Input: part model. Units: mm. Frame: model coordinates. Face numbers are marked on the shaded views. A direction names the side the tool comes from. Coordinates: 2 decimals unless noted, no trailing zeros. Write each loop counter-clockwise with the first axis right and the second up, starting at its lowest first coordinate (ties: lowest second). Pieces come first, ordered by that corner, then holes. Notation, with made-up numbers: (71.25, 66.25) -> (107.25, 66.25) arc R9 ccw to (107.25, 81.25) -> close; hole circle Ø8 at (-33.75, -35.5). An arc over 180 degrees is marked (long way). Use one line per item in the form item = value. Start each with the question number.
(1) Cut plane C-C on x = 78. Return the cut outline in (y, z), plus the area to 3 significant figures.
(2) Pull-direction query (Y, two-part tool) for the marked faces 6, 7 and 8; classes: released by +Y, released by -Y, zero draft, split by the parting line, or undercut.
(3) Set-up query: the marked faces 1, 2, 3, 4 and 5. Return all of +Z, -Z, +X, -X, +Y, -Y with unobstructed straight access to the full face (end or side cutting, diameter ignored); none if empty.
(4) Cut plane B-B on y = 0. Return the cut outline in (x, z), plus the area to 3 significant figures.
(5) Ray query, line 1 along X through (y, z) = (-13.5, 16); line 2 along X through (y, z) = (11, 10.5); line 3 along Y through (x, z) = (27, -6.5). Return the intervals inside material, ascending.
(6) First-contact query: pin 1 (6 mm diameter, centred on x = 101, y = -14.5, fed in from -Z); pin 2 (10 mm diameter, centred on x = 47.5, y = 1, fed in from +Z); pin 3 (1.5 mm diameter, centred on x = 8, z = 0.5, fed in from -Y); pin 4 (19.5 mm diameter, centred on x = 62.5, z = -3, fed in from +Y). Flat tips, straight axial feed; report the tip coordinate or a pass-through.
(7) Cut plane D-D on y = -7. Return the cut outline in (x, z), plus the area to 3 significant figures.
(8) Cut plane A-A on z = -1.5. Return the cut outline in (x, y), plus the area to 3 significant figures.
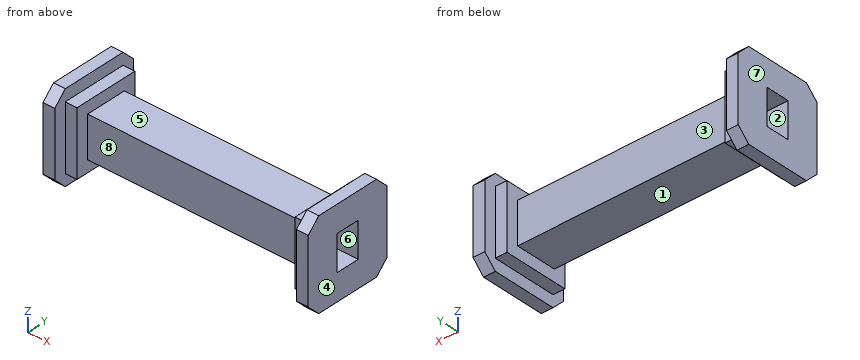
```python
from build123d import *

# Parameters (mm, degrees)
SKETCH1_W           = 38.1
SKETCH1_H           = 38.1
BOSS_EXTRUDE1_DEPTH = 114.3
CUT_EXTRUDE1_START  = -5.08
SKETCH3_W           = 38.1
SKETCH3_H           = 38.1
SKETCH3_W_2         = 27.94
SKETCH3_H_2         = 27.94
CUT_EXTRUDE1_DEPTH  = 104.14
CUT_EXTRUDE2_START  = -93.98
SKETCH4_W           = 38.1
SKETCH4_H           = 38.1
SKETCH4_W_2         = 17.78
SKETCH4_H_2         = 17.78
CUT_EXTRUDE2_DEPTH  = 93.98
SKETCH5_W           = 15.24
SKETCH5_H           = 10.16
CUT_EXTRUDE3_DEPTH  = 118.432086757
CHAMFER1_SIZE       = 5.08


with BuildPart() as part:
    # Sketch1 → Boss-Extrude1 (new body)
    with BuildSketch(Plane(origin=(0, 0, 0), x_dir=(0, 0, -1), z_dir=(1, 0, 0))):
        Rectangle(SKETCH1_W, SKETCH1_H)
    extrude(amount=BOSS_EXTRUDE1_DEPTH)

    # Sketch3 → Cut-Extrude1 (cut)
    with BuildSketch(Plane.ZY.offset(CUT_EXTRUDE1_START)):
        Rectangle(SKETCH3_W, SKETCH3_H)
        Rectangle(SKETCH3_W_2, SKETCH3_H_2, mode=Mode.SUBTRACT)
    extrude(amount=-CUT_EXTRUDE1_DEPTH, mode=Mode.SUBTRACT)

    # Sketch4 → Cut-Extrude2 (cut)
    with BuildSketch(Plane.ZY.offset(-10.16).offset(CUT_EXTRUDE2_START)):
        Rectangle(SKETCH4_W, SKETCH4_H)
        Rectangle(SKETCH4_W_2, SKETCH4_H_2, mode=Mode.SUBTRACT)
    extrude(amount=CUT_EXTRUDE2_DEPTH, mode=Mode.SUBTRACT)

    # Sketch5 → Cut-Extrude3 (cut, through all)
    with BuildSketch(Plane.ZY):
        Rectangle(SKETCH5_W, SKETCH5_H)
    extrude(amount=-CUT_EXTRUDE3_DEPTH, mode=Mode.SUBTRACT)

    # Chamfer1
    chamfer1_edges = [part.edges().sort_by_distance(p)[0] for p in [
        (2.54, -19.05, -19.05),
        (2.54, -19.05, 19.05),
        (2.54, 19.05, 19.05),
        (2.54, 19.05, -19.05),
        (111.76, -19.05, -19.05),
        (111.76, -19.05, 19.05),
        (111.76, 19.05, 19.05),
        (111.76, 19.05, -19.05),
    ]]
    chamfer(chamfer1_edges, length=CHAMFER1_SIZE)


solid = part.part
```
Values:
q1.outline = (-8.89, -8.89) -> (8.89, -8.89) -> (8.89, 8.89) -> (-8.89, 8.89) -> close; hole (-5.08, -7.62) -> (5.08, -7.62) -> (5.08, 7.62) -> (-5.08, 7.62) -> close
q1.area = 161 mm2
q2.face_6 = undercut
q2.face_7 = zero draft
q2.face_8 = released by -Y
q3.face_1 = -Z, +Y, -Y
q3.face_2 = +X, -X
q3.face_3 = +Z, -Z, +Y
q3.face_4 = +Z, -Z, +X, +Y, -Y
q3.face_5 = +Z, +Y, -Y
q4.outline = (0, -19.05) -> (5.08, -19.05) -> (5.08, -13.97) -> (10.16, -13.97) -> (10.16, -8.89) -> (104.14, -8.89) -> (104.14, -13.97) -> (109.22, -13.97) -> (109.22, -19.05) -> (114.3, -19.05) -> (114.3, -7.62) -> (0, -7.62) -> close; (0, 7.62) -> (114.3, 7.62) -> (114.3, 19.05) -> (109.22, 19.05) -> (109.22, 13.97) -> (104.14, 13.97) -> (104.14, 8.89) -> (10.16, 8.89) -> (10.16, 13.97) -> (5.08, 13.97) -> (5.08, 19.05) -> (0, 19.05) -> close
q4.area = 600 mm2
q5.line_1 = 0 to 5.08, 109.22 to 114.3
q5.line_2 = 0 to 10.16, 104.14 to 114.3
q5.line_3 = -8.89 to -5.08, 5.08 to 8.89
q6.pin_1 = through
q6.pin_2 = 8.89
q6.pin_3 = -13.97
q6.pin_4 = 8.89
q7.outline = (0, -19.05) -> (5.08, -19.05) -> (5.08, -13.97) -> (10.16, -13.97) -> (10.16, -8.89) -> (104.14, -8.89) -> (104.14, -13.97) -> (109.22, -13.97) -> (109.22, -19.05) -> (114.3, -19.05) -> (114.3, 19.05) -> (109.22, 19.05) -> (109.22, 13.97) -> (104.14, 13.97) -> (104.14, 8.89) -> (10.16, 8.89) -> (10.16, 13.97) -> (5.08, 13.97) -> (5.08, 19.05) -> (0, 19.05) -> close
q7.area = 2,340 mm2
q8.outline = (0, -19.05) -> (5.08, -19.05) -> (5.08, -13.97) -> (10.16, -13.97) -> (10.16, -8.89) -> (104.14, -8.89) -> (104.14, -13.97) -> (109.22, -13.97) -> (109.22, -19.05) -> (114.3, -19.05) -> (114.3, -5.08) -> (0, -5.08) -> close; (0, 5.08) -> (114.3, 5.08) -> (114.3, 19.05) -> (109.22, 19.05) -> (109.22, 13.97) -> (104.14, 13.97) -> (104.14, 8.89) -> (10.16, 8.89) -> (10.16, 13.97) -> (5.08, 13.97) -> (5.08, 19.05) -> (0, 19.05) -> close
q8.area = 1,180 mm2
